CAD build for the part. Positions are in the model's coordinates, mm. Face numbers are marked on the shaded views. A direction names the side the tool comes from. Round coordinates to 2 decimals unless told otherwise and drop trailing zeros. Write each loop counter-clockwise with the first axis right and the second up, starting at its lowest first coordinate (ties: lowest second). Pieces come first, ordered by that corner, then holes. Notation, with made-up numbers: (0.5, 34.25) - (57.5, 34.25) arc R15 cw to (57.5, 41.25) - close; hole circle Ø6 at (-36, 19.25). An arc over 180 degrees is marked (long way). Use one line per item in the form item = value. Start each with the question number.
Item 1: Tool access for the marked faces 1, 2 and 3: list every direction of +Z, -Z, +X, -X, +Y, -Y with a clear straight run to the whole face (end or side of a thin tool).
Item 2: Band-saw the part on A-A, the plane y = 38. List the corners of the cut face in (x, z).
Item 3: Band-saw the part on D-D, the plane y = 6. List the corners of the cut face in (x, z).
Item 4: Pin check, flat tips, straight feed: pin 1 (2.5 mm diameter, centred on x = 16.5, z = 0.5, fed in from -Y); pin 2 (0.5 mm diameter, centred on y = 16.5, z = -0.5, fed in from -X); pin 3 (0.5 mm diameter, centred on y = 17.5, z = -0.5, fed in from +X). Stop position of each tip, or through.
Item 5: Band-saw the part on B-B, the plane x = 48. List the corners of the cut face in (y, z), and give its area (4 significant figures).
Item 6: Band-saw the part on C-C, the plane z = 1.4. List the corners of the cut face in (x, y), and give its area (3 significant figures).
Item 7: Drill centre lines: L1, parallel to X at y = 20, z = 1.65; L2, parallel to Y at x = 61, z = 2.7; L3, parallel to Z at x = 63, y = 25.5. Where is each one in solid material? Low to high.
Item 8: Pull direction X, two halves, no side cores. Call the marked faces 4 and 5: +X half, -X half, draft (parallel to the pull), parting line (faces both ways), or undercut.
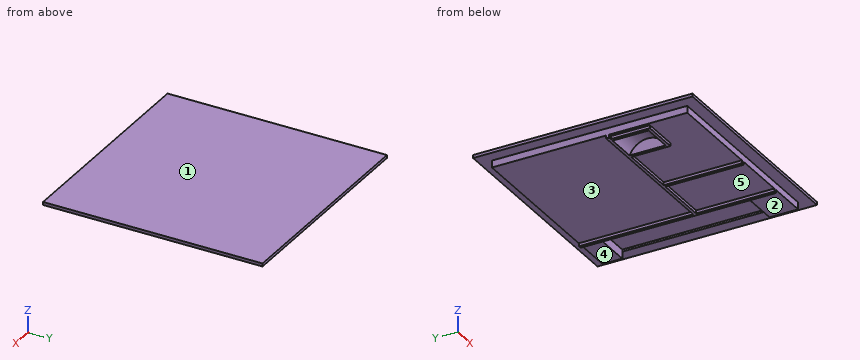
Autodesk Inventor part; units mm, degrees
ref_plane "YZ Plane" through (0, 0, 0) normal (1, 0, 0) x (0, 1, 0)
ref_plane "XZ Plane" through (0, 0, 0) normal (0, 1, 0) x (-1, 0, 0)
ref_plane "XY Plane" through (0, 0, 0) normal (0, 0, 1) x (1, 0, 0)
sketch "Sketch1" plane through (0, 0, 0) normal (0, 0, 1) x (1, 0, 0)
  line L0 (0, 0) -> (65, 0)
  line L1 (65, 0) -> (65, 65)
  line L2 (65, 65) -> (0, 65)
  line L3 (0, 65) -> (0, 0)
  dimension "d0" = 65
  dimension "d1" = 65
extrude "Extrusion1" add sketch "Sketch1" along normal blind 2.3
sketch "Sketch2" plane through (0, 0, 2.3) normal (0, 0, 1) x (1, 0, 0)
  line L0 (-4, 69) -> (69, 69)
  line L1 (69, 69) -> (69, -4)
  line L2 (69, -4) -> (-4, -4)
  line L3 (-4, -4) -> (-4, 69)
  point P0 (0, 0)
  point P1 (0, 65)
  point P2 (65, 0)
extrude "Extrusion2" add sketch "Sketch2" along normal blind 1
sketch "Sketch3" plane through (0, 0, 0) normal (0, 0, -1) x (-1, 0, 0)
  line L0 (0, 0) -> (-65, 0)
  line L1 (0, 65) -> (0, 0)
  line L2 (-65, 0) -> (-65, 65)
  line L3 (-52, 65) -> (-52, 26)
  line L4 (-52, 26) -> (0, 26)
  line L5 (-51, 27) -> (-51, 65)
  line L6 (-51, 65) -> (-52, 65)
  line L7 (0, 65) -> (-1, 65)
  line L8 (-51, 27) -> (0, 27)
  point P0 (0, 26)
extrude "Extrusion5" add sketch "Sketch3" along normal blind 1
sketch "Sketch6" plane through (0, 0, 0) normal (0, 0, -1) x (-1, 0, 0)
  line L0 (-65, 65) -> (-52, 65)
  line L1 (-65, 55.5) -> (-52, 55.5)
  line L2 (-52, 26) -> (-52, 65)
  line L3 (-52, 55.5) -> (-52, 9.5)
  line L4 (-52, 9.5) -> (-65, 9.5)
  line L5 (-65, 9.5) -> (-65, 55.5)
  line L6 (-65, 0) -> (-65, 65)
  point P0 (0, 0)
  dimension "d23" = 46
extrude "Extrusion6" cut sketch "Sketch6" against normal blind 3 contours L1 L2 L3 L4 L5
sketch "Sketch7" plane through (0, 0, 0) normal (0, 0, -1) x (-1, 0, 0)
  line L0 (-65, 9.5) -> (-65, 55.5)
  line L1 (-52, 55.5) -> (-52, 65)
  line L2 (-52, 55.5) -> (-65, 55.5)
  line L3 (-65, 55.5) -> (-65, 58.5)
  line L4 (-65, 58.5) -> (-52, 58.5)
  line L5 (-52, 58.5) -> (-52, 55.5)
  point P0 (0, 0)
extrude "Extrusion7" cut sketch "Sketch7" against normal blind 3
sketch "Sketch8" plane through (0, 0, 0) normal (0, 0, -1) x (-1, 0, 0)
  line L0 (-52, 26) -> (-52, 9.5)
  line L1 (-52, 26) -> (-52, 0)
  line L2 (-52, 26) -> (-51, 26)
  line L3 (-51, 26) -> (-51, 0)
  line L4 (0, 0) -> (-65, 0)
  line L5 (-52, 0) -> (-51, 0)
  line L6 (-51, 26) -> (-33, 26)
  line L7 (0, 26) -> (-52, 26)
  line L8 (-33, 26) -> (-33, 0)
  line L9 (-33, 0) -> (-32, 0)
  line L10 (-32, 0) -> (-32, 26)
  line L11 (-32, 26) -> (-33, 26)
  dimension "d32" = 1
extrude "Extrusion8" add sketch "Sketch8" along normal blind 1 contours L2 L3 L4 L1 L0 | L7 L10 L4 L8
sketch "Sketch9" plane through (0, 0, 0) normal (0, 0, -1) x (-1, 0, 0)
  line L0 (0, 26) -> (0, 0)
  line L1 (0, 26) -> (-32, 26)
  line L2 (-2, 26) -> (-12, 26)
  line L3 (-12, 26) -> (-12, 14)
  line L4 (-12, 14) -> (-2, 14)
  line L5 (-2, 14) -> (-2, 26)
  line L6 (-1, 13) -> (-13, 13)
  line L7 (-13, 13) -> (-13, 26)
  line L8 (-1, 13) -> (-1, 26)
  line L9 (-12, 26) -> (-13, 26)
  line L10 (-2, 26) -> (-1, 26)
  dimension "d35" = 2
  dimension "d36" = 10
  dimension "d37" = 12
extrude "Extrusion9" add sketch "Sketch9" along normal blind 1 contours L8 L6 L7 L1 L3 L4 L5
sketch "Sketch12" plane through (0, 0, 0) normal (0, 0, -1) x (-1, 0, 0)
  line L0 (-12, 14) -> (-2, 14)
  line L1 (-12, 26) -> (-2, 26)
  line L2 (-12, 14) -> (-2, 14)
  line L3 (-2, 14) -> (-2, 26)
  line L4 (-2, 26) -> (-12, 26)
  line L5 (-12, 26) -> (-12, 14)
  point P0 (0, 0)
extrude "Extrusion11" cut sketch "Sketch12" against normal blind 3
fillet "Fillet1" radius 6.5 2 edges at (7, 14, 3) (7, 26, 3)
properties part number "CaseBottom"
Determined:
q1.face_1 = +Z, +X, -X, +Y, -Y
q1.face_2 = -Z, +X, +Y, -Y
q1.face_3 = -Z, -X, +Y
q2.outline = (-4, 2.3) - (0, 2.3) - (0, 0) - (51, 0) - (51, -1) - (52, -1) - (52, 3) - (65, 3) - (65, 2.3) - (69, 2.3) - (69, 3.3) - (-4, 3.3) - close
q3.outline = (-4, 2.3) - (0, 2.3) - (0, 0) - (32, 0) - (32, -1) - (33, -1) - (33, 0) - (51, 0) - (51, -1) - (52, -1) - (52, 0) - (65, 0) - (65, 2.3) - (69, 2.3) - (69, 3.3) - (-4, 3.3) - close
q4.pin_1 = 0
q4.pin_2 = 1
q4.pin_3 = 52
q5.outline = (-4, 2.3) - (0, 2.3) - (0, 0) - (26, 0) - (26, -1) - (27, -1) - (27, 0) - (65, 0) - (65, 2.3) - (69, 2.3) - (69, 3.3) - (-4, 3.3) - close
q5.area = 223.5 mm²
q6.outline = (0, 0) - (65, 0) - (65, 9.5) - (52, 9.5) - (52, 58.5) - (65, 58.5) - (65, 65) - (0, 65) - close; hole (2, 15.73) - (12, 15.73) - (12, 24.27) - (2, 24.27) - close
q6.area = 3,500 mm²
q7.L1 = 0 to 2, 12 to 52
q7.L2 = -4 to 9.5, 58.5 to 69
q7.L3 = 3 to 3.3
q8.face_4 = draft
q8.face_5 = undercut
